from build123d import *

# Parameters (mm, degrees)
SKETCH1_W           = 19.05
SKETCH1_H           = 19.05
SKETCH1_W_2         = 12.7
SKETCH1_H_2         = 12.7
BOSS_EXTRUDE1_DEPTH = 69.85
CUT_EXTRUDE1_DEPTH  = 74.025
SKETCH3_R           = 5.55625
CUT_EXTRUDE2_DEPTH  = 74.025
SKETCH4_R           = 2.54
CUT_EXTRUDE3_DEPTH  = 74.025


with BuildPart() as part:
    # Sketch1 → Boss-Extrude1 (new, symmetric)
    with BuildSketch(Plane.XY):
        Rectangle(SKETCH1_W, SKETCH1_H)
        Rectangle(SKETCH1_W_2, SKETCH1_H_2, mode=Mode.SUBTRACT)
    extrude(amount=BOSS_EXTRUDE1_DEPTH, both=True)

    # Sketch2 → Cut-Extrude1 (cut, through all)
    with BuildSketch(Plane(origin=(9.525, 0, 0), x_dir=(0, 0, -1), z_dir=(1, 0, 0))):
        Polygon((-69.85, 9.525), (-61.959231637, -9.525), (-69.85, -9.525), align=None)
    extrude(amount=-CUT_EXTRUDE1_DEPTH, mode=Mode.SUBTRACT)

    # Sketch3 → Cut-Extrude2 (cut, through all)
    with BuildSketch(Plane(origin=(9.525, 0, 0), x_dir=(0, 0, -1), z_dir=(1, 0, 0))):
        with Locations((52.340768363, 0)):
            Circle(SKETCH3_R)
    extrude(amount=-CUT_EXTRUDE2_DEPTH, mode=Mode.SUBTRACT)

    # Sketch4 → Cut-Extrude3 (cut, through all)
    with BuildSketch(Plane(origin=(0, 9.525, 0), x_dir=(1, 0, 0), z_dir=(0, 1, 0))):
        with Locations(Location((0, 52.340768363, 0), (0, 0, 270))):
            Circle(SKETCH4_R)
    extrude(amount=-CUT_EXTRUDE3_DEPTH, mode=Mode.SUBTRACT)


solid = part.part
The listing builds one solid part. Answer for the finished solid, in the listing's coordinates (mm). A direction names the side the tool comes from. Coordinates: 2 decimals unless noted, no trailing zeros. Order: outer loops, then holes, each group sorted by start corner. A loop starts at its lowest first (then second) coordinate and runs counter-clockwise, first axis right, second up.
Q1. Which of the six approach directions +Z, -Z, +X, -X, +Y, -Y give full straight-line access (tool end or side, diameter ignored) to faces 1 (the face through (-9.525, 0, 1)), 2 (the face through (0, -6.35, -2))?
Q2. A cutting plane is placed at C-C, the plane y = 2. Write down the section's boundary in (x, z) (3 decimals), and give its area (3 significant figures).
Q3. Given P1, Ø4, axis at x = 0, z = -52.34, coming from the +Y side; P2, Ø2, axis at x = 6.5, y = -4, coming from the +Z side; P3, Ø6, axis at x = -7.5, y = -1.5, coming from the +Z side, each flat-ended and moving along its own axis, determine where each tip first touches the part or whether it passes through.
Q4. A cutting plane is placed at A-A, the plane x = 3.75. Write down the section's boundary in (y, z) (3 decimals).
Q5. For a pull along X with two mould halves and no side action, classify faces 3 (the face through (7.96, 0.24, -46.79)), 4 (the face through (9.525, 0, 1)), 5 (the face through (-6.35, 0, 0)) as pulls with the +X half, pulls with the -X half, needs draft (parallel to the pull), parting line crosses it, or undercut.
Q6. Consider line 1 (X direction, y = -6.25, z = -34.5) (3 decimals); line 2 (Z direction, x = 8.25, y = -8.25). Determine where each line is inside the solid, lowest interval first.
Q7. A cutting plane is placed at D-D, the plane y = -3.75. Write down the section's boundary in (x, z) (3 decimals).
Q8. A cutting plane is placed at B-B, the plane z = -11.5. Write down the section's boundary in (x, y) (3 decimals).
Answers follow:
1. face 1: +Z, -Z, -X, +Y, -Y
1. face 2: +Z, -Z
2. outline: (-9.525, -69.85) - (-6.35, -69.85) - (-6.35, -57.525) - (-9.525, -57.525) - close; (-9.525, -47.157) - (-6.35, -47.157) - (-6.35, 66.733) - (-9.525, 66.733) - close; (6.35, -69.85) - (9.525, -69.85) - (9.525, -57.525) - (6.35, -57.525) - close; (6.35, -47.157) - (9.525, -47.157) - (9.525, 66.733) - (6.35, 66.733) - close
2. area: 801 mm2
3. P1: passes through
3. P2: stops at z = 64.66
3. P3: stops at z = 66.53
4. outline: (-9.525, -69.85) - (-6.35, -69.85) - (-6.35, 63.274) - (-9.525, 61.959) - close; (6.35, -69.85) - (9.525, -69.85) - (9.525, 69.85) - (6.35, 68.535) - close
5. face 3: needs draft
5. face 4: pulls with the +X half
5. face 5: undercut
6. line 1: x = -9.525 to -6.35, 6.35 to 9.525
6. line 2: z = -69.85 to 62.49
7. outline: (-9.525, -69.85) - (-6.35, -69.85) - (-6.35, -56.441) - (-9.525, -56.441) - close; (-9.525, -48.241) - (-6.35, -48.241) - (-6.35, 64.351) - (-9.525, 64.351) - close; (6.35, -69.85) - (9.525, -69.85) - (9.525, -56.441) - (6.35, -56.441) - close; (6.35, -48.241) - (9.525, -48.241) - (9.525, 64.351) - (6.35, 64.351) - close
8. outline: (-9.525, -9.525) - (9.525, -9.525) - (9.525, 9.525) - (-9.525, 9.525) - close; hole (-6.35, -6.35) - (6.35, -6.35) - (6.35, 6.35) - (-6.35, 6.35) - close
